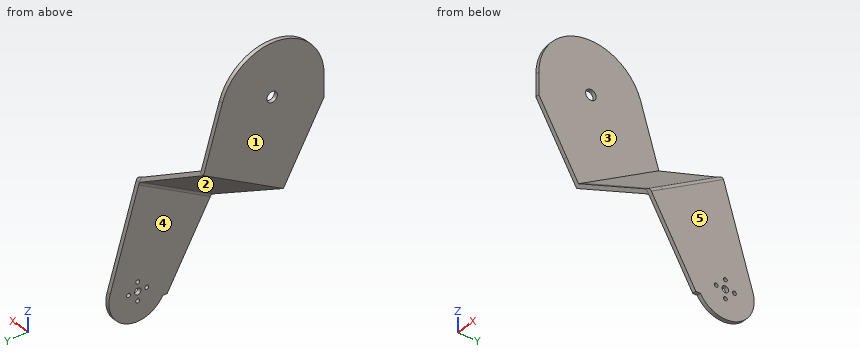
from build123d import *

# Parameters (mm, degrees)
SKETCH_2_R           = 3
SKETCH_2_R_2         = 1.5
SKETCH_2_R_3         = 2.5
EXTRUDE_1_DEPTH      = 3
EXTRUDE_2_DEPTH      = 196
SKETCH_5_R           = 8
CUT_EXTRUDE_1_DEPTH  = 10
SKETCH_6_R           = 4.05
CUT_EXTRUDE_2_DEPTH  = 10
SKETCH_8_R           = 40
EXTRUDE_3_DEPTH      = 3
EXTRUDE_START        = -61
EXTRUDE_4_DEPTH      = 64
EXTRUDE_5_DEPTH      = 3
EXTRUDE_START_2      = -3
EXTRUDE_14_DEPTH     = 3
EXTRUDE_15_DEPTH     = 3
SKETCH_16_R          = 40
EXTRUDE_16_DEPTH     = 3
CUT_EXTRUDE_START    = -20
CUT_EXTRUDE_5_DEPTH  = 20
CUT_EXTRUDE_6_DEPTH  = 20
CUT_EXTRUDE_7_DEPTH  = 3
FILLET_3_R           = 3
FILLET_4_R           = 3
FILLET_5_R           = 3
FILLET_6_R           = 3
SKETCH_22_R          = 7.75
CUT_EXTRUDE_8_DEPTH  = 10
SKETCH_23_R          = 4.05
CUT_EXTRUDE_9_DEPTH  = 10
CUT_EXTRUDE_10_DEPTH = 10
SKETCH_25_W          = 514.702896461
SKETCH_25_H          = 285.568662858
CUT_EXTRUDE_11_DEPTH = 80


# Some blends are built 0.0001 mm under size
with BuildPart() as part:
    # Sketch 2 → Extrude 1 (new body)
    with BuildSketch(Plane(origin=(0, 0, 0), x_dir=(0, 0, -1), z_dir=(1, 0, 0))):
        with BuildLine():
            Line((138.514809283, 84.200667909), (-11.70063651, 38.25042621))
            ThreePointArc((-11.70063651, 38.25042621), (-39.560188627, -5.915359313), (0, -40))
            Line((0, -40), (16.710190716, -40))
            Line((16.710190716, -40), (156.071648789, 40.329376559))
            Line((156.071648789, 40.329376559), (156.071648789, 43.792069046))
            ThreePointArc((156.071648789, 43.792069046), (165.334026038, 71.834783727), (138.514809283, 84.200667909))
        make_face()
        Circle(SKETCH_2_R, mode=Mode.SUBTRACT)
        with Locations((145, 70)):
            Circle(SKETCH_2_R_2, mode=Mode.SUBTRACT)
        with Locations((138, 63)):
            Circle(SKETCH_2_R_2, mode=Mode.SUBTRACT)
        with Locations((145, 56)):
            Circle(SKETCH_2_R_2, mode=Mode.SUBTRACT)
        with Locations((145, 63)):
            Circle(SKETCH_2_R_3, mode=Mode.SUBTRACT)
        with Locations((152, 63)):
            Circle(SKETCH_2_R_2, mode=Mode.SUBTRACT)
    extrude_1 = extrude(amount=EXTRUDE_1_DEPTH)

    # Sketch 4 → Extrude 2 (add)
    with BuildSketch(Plane(origin=(3, 0, 0), x_dir=(0, 0, -1), z_dir=(1, 0, 0))):
        with BuildLine():
            Line((0, -40), (16.710190716, -40))
            Line((16.710190716, -40), (156.071648789, 40.329376559))
            Line((156.071648789, 40.329376559), (156.071648789, 43.792069046))
            Line((156.071648789, 43.792069046), (19.975563357, -34.655113166))
            ThreePointArc((19.975563357, -34.655113166), (10.339136167, -38.640681455), (0, -40))
        make_face()
    extrude(amount=EXTRUDE_2_DEPTH)

    # Mirror 2: Extrude 1 across plane
    add(extrude_1.mirror(Plane(origin=(101, 0, 0), x_dir=(0, 0, 1), z_dir=(1, 0, 0))))

    # Sketch 5 → Cut-Extrude 1 (cut)
    with BuildSketch(Plane(origin=(202, 0, 0), x_dir=(0, 0, -1), z_dir=(1, 0, 0))):
        Circle(SKETCH_5_R)
    extrude(amount=-CUT_EXTRUDE_1_DEPTH, mode=Mode.SUBTRACT)

    # Sketch 6 → Cut-Extrude 2 (cut)
    with BuildSketch(Plane.ZY):
        Circle(SKETCH_6_R)
    extrude(amount=-CUT_EXTRUDE_2_DEPTH, mode=Mode.SUBTRACT)

    # Sketch 9 → Extrude 4 (add)
    with BuildSketch(Plane(origin=(251, 0, 0), x_dir=(0, 0, -1), z_dir=(1, 0, 0)).offset(EXTRUDE_START)):
        with BuildLine():
            Line((0, -40), (16.710190716, -40))
            Line((16.710190716, -40), (53.747942483, -18.651059269))
            Line((53.747942483, -18.651059269), (52.249775231, -16.051925781))
            Line((52.249775231, -16.051925781), (19.975563357, -34.655113166))
            ThreePointArc((19.975563357, -34.655113166), (10.339136167, -38.640681455), (0, -40))
        make_face()
    extrude_4 = extrude(amount=EXTRUDE_4_DEPTH)

    # Sketch 10 → Extrude 5 (add)
    with BuildSketch(Plane(origin=(0, -37.254246654, -21.473730609), x_dir=(1, 0, 0), z_dir=(0, -0.8663778291595938, -0.49938908392225567))):
        Polygon((254, -37.251890328), (254, -57.251890328), (202, -87.274104325), (202, -37.251890328), align=None)
    extrude_5 = extrude(amount=-EXTRUDE_5_DEPTH)



with BuildPart() as body_2:
    # Sketch 8 → Extrude 3 (new body)
    with BuildSketch(Plane(origin=(251, 0, 0), x_dir=(0, 0, -1), z_dir=(1, 0, 0))):
        Circle(SKETCH_8_R)
    extrude(amount=EXTRUDE_3_DEPTH)


with BuildPart() as part_1:
    add(part.part)

    add(body_2.part)  # Extrude 14 merges body 2
    # Sketch 14 → Extrude 14 (add)
    with BuildSketch(Plane(origin=(254, 0, 0), x_dir=(0, 0, -1), z_dir=(1, 0, 0)).offset(EXTRUDE_START_2)):
        with BuildLine():
            Line((-11.70063651, 38.25042621), (35.679778873, 52.743886101))
            Line((35.679778873, 52.743886101), (69.577331814, -6.064144103))
            Line((69.577331814, -6.064144103), (19.975563357, -34.655113166))
            ThreePointArc((19.975563357, -34.655113166), (36.686823541, 15.939792297), (-11.70063651, 38.25042621))
        make_face()
    extrude_14 = extrude(amount=EXTRUDE_14_DEPTH)

    # Sketch 15 → Extrude 15 (add)
    with BuildSketch(Plane(origin=(88.290795719, 76.368648195, -132.490087928), x_dir=(-0.8660254037844362, 0.24969454196113003, -0.4331889145798008), z_dir=(0.5000000000000044, 0.4324836330493111, -0.7503052093278204))):
        Polygon((-191.344507397, -43), (-191.344507397, 27.878041456), (-131.300079402, 20.97393325), (-131.300079402, -43), align=None)
    extrude_15 = extrude(amount=-EXTRUDE_15_DEPTH)

    # Mirror 8: Extrude 15 across plane
    add(extrude_15.mirror(Plane(origin=(101, 0, 0), x_dir=(0, 0, 1), z_dir=(1, 0, 0))))

    # Mirror 10: Extrude 5 across plane
    add(extrude_5.mirror(Plane(origin=(101, 0, 0), x_dir=(0, 0, 1), z_dir=(1, 0, 0))))

    # Mirror 11: Extrude 4 across plane
    add(extrude_4.mirror(Plane(origin=(101, 0, 0), x_dir=(0, 0, 1), z_dir=(1, 0, 0))))

    # Mirror 12: Extrude 14 across plane
    add(extrude_14.mirror(Plane(origin=(101, 0, 0), x_dir=(0, 0, 1), z_dir=(1, 0, 0))))

    # Sketch 16 → Extrude 16 (add)
    with BuildSketch(Plane.ZY.offset(52)):
        Circle(SKETCH_16_R)
    extrude(amount=-EXTRUDE_16_DEPTH)

    # Sketch 17 → Cut-Extrude 5 (cut)
    with BuildSketch(Plane(origin=(202, 0, 0), x_dir=(0, 0, -1), z_dir=(1, 0, 0)).offset(CUT_EXTRUDE_START)):
        with BuildLine():
            Line((-11.120326036, 38.423148607), (61.739147636, 60.715331959))
            Line((61.739147636, 60.715331959), (65.138195736, 61.755085767))
            Line((65.138195736, 61.755085767), (62.037518083, 60.197696416))
            Line((62.037518083, 60.197696416), (92.586691567, 7.198687311))
            Line((92.586691567, 7.198687311), (19.975563357, -34.655113166))
            ThreePointArc((19.975563357, -34.655113166), (-36.806411031, -15.66167638), (-11.120326036, 38.423148607))
        make_face()
    extrude(amount=CUT_EXTRUDE_5_DEPTH, mode=Mode.SUBTRACT)


with BuildPart() as cut_extrude_5_piece_1:
    # of the separate pieces the step leaves, piece 1, a body of its own (cut_extrude_5_pieces)
    add(part_1.part.solids().sort_by_distance((0, 43.792069046, -156.071648789))[0])

    # Sketch 21 → Cut-Extrude 7 (cut)
    with BuildSketch(Plane(origin=(3, 0, 0), x_dir=(0, 0, -1), z_dir=(1, 0, 0))):
        with BuildLine():
            Line((92.586691567, 7.198687311), (62.037518083, 60.197696416))
            Line((62.037518083, 60.197696416), (65.138195736, 61.755085767))
            Line((65.138195736, 61.755085767), (61.739147636, 60.715331959))
            Line((61.739147636, 60.715331959), (-11.70063651, 38.25042621))
            ThreePointArc((-11.70063651, 38.25042621), (-36.686823541, -15.939792297), (19.975563357, -34.655113166))
            Line((19.975563357, -34.655113166), (92.586691567, 7.198687311))
        make_face()
    extrude(amount=-CUT_EXTRUDE_7_DEPTH, mode=Mode.SUBTRACT)

    # Fillet 3
    fillet_3_edges = [cut_extrude_5_piece_1.edges().sort_by_distance(p)[0] for p in [
        (3, 33.698191863, -77.312104825),
    ]]
    fillet(fillet_3_edges, radius=FILLET_3_R - 0.0001)  # a hair under: the kernel refuses the full size

    # Fillet 4
    fillet_4_edges = [cut_extrude_5_piece_1.edges().sort_by_distance(p)[0] for p in [
        (199, 33.698191863, -77.312104825),
    ]]
    fillet(fillet_4_edges, radius=FILLET_4_R - 0.0001)  # a hair under: the kernel refuses the full size

    # Fillet 5
    # the kernel refuses this fillet: 3 mm, written as the material it adds along each edge
    with BuildSketch(Plane(origin=(202, 65.506611814, -62.97577757), x_dir=(0, 0.49938908392225534, -0.8663778291595939), z_dir=(0, -0.866377829159594, -0.4993890839222554))) as fillet_5_piece_1_section:
        with BuildLine():
            CenterArc((FILLET_5_R * 0.57735026919, FILLET_5_R), FILLET_5_R, 210, 60)
            Line((-FILLET_5_R * 0.288675134595, FILLET_5_R * 0.5), (0, 0))
            Line((0, 0), (FILLET_5_R * 0.57735026919, 0))
        make_face()
    fillet_5_piece_1 = extrude(amount=68.304060269, mode=Mode.PRIVATE)
    fillet_5_piece_1 = split(fillet_5_piece_1, bisect_by=Plane(origin=(202.325553984, 63.906694987, -72.171998522), z_dir=(0, -0.9562606552534866, -0.2925159127537726)), keep=Keep.TOP, mode=Mode.PRIVATE)
    fillet_5_piece_1 = split(fillet_5_piece_1, bisect_by=Plane(origin=(199.177617764, 62.412552566, -67.072312804), z_dir=(0.09892666816624712, -0.8892295154916122, -0.44663674625368427)), keep=Keep.TOP, mode=Mode.PRIVATE)
    add(fillet_5_piece_1)

    # Fillet 6
    # the kernel refuses this fillet: 3 mm, written as the material it adds along each edge
    with BuildSketch(Plane(origin=(0, 6.329488355, -97.086079656), x_dir=(2.017234182721707e-14, 0.49938908392225534, -0.8663778291595939), z_dir=(0, 0.8663778291595939, 0.4993890839222554))) as fillet_6_piece_1_section:
        with BuildLine():
            CenterArc((FILLET_6_R * 0.57735026919, FILLET_6_R), FILLET_6_R, 210, 60)
            Line((-FILLET_6_R * 0.288675134595, FILLET_6_R * 0.5), (0, 0))
            Line((0, 0), (FILLET_6_R * 0.57735026919, 0))
        make_face()
    fillet_6_piece_1 = extrude(amount=68.304060269, mode=Mode.PRIVATE)
    fillet_6_piece_1 = split(fillet_6_piece_1, bisect_by=Plane(origin=(-0.325553984, 63.906694987, -72.171998522), z_dir=(0, -0.9562606552534866, -0.2925159127537726)), keep=Keep.TOP, mode=Mode.PRIVATE)
    fillet_6_piece_1 = split(fillet_6_piece_1, bisect_by=Plane(origin=(2.822382236, 62.412552566, -67.072312804), z_dir=(-0.09892666816624712, -0.8892295154916122, -0.44663674625368427)), keep=Keep.TOP, mode=Mode.PRIVATE)
    add(fillet_6_piece_1)

    # Sketch 22 → Cut-Extrude 8 (cut)
    with BuildSketch(Plane(origin=(254, 0, 0), x_dir=(0, 0, -1), z_dir=(1, 0, 0))):
        Circle(SKETCH_22_R)
    extrude(amount=-CUT_EXTRUDE_8_DEPTH, mode=Mode.SUBTRACT)

    # Sketch 23 → Cut-Extrude 9 (cut)
    with BuildSketch(Plane.ZY.offset(52)):
        Circle(SKETCH_23_R)
    extrude(amount=-CUT_EXTRUDE_9_DEPTH, mode=Mode.SUBTRACT)

    # Sketch 24 → Cut-Extrude 10 (cut)
    with BuildSketch(Plane(origin=(0, -37.254246654, -21.473730609), x_dir=(1, 0, 0), z_dir=(0, -0.8663778291595938, -0.49938908392225567))):
        with BuildLine():
            Line((-49, 40), (-49, -55.51983952))
            Line((-49, -55.51983952), (0, -83.81000271))
            ThreePointArc((0, -83.81000271), (2.121320344, -84.688682367), (3, -86.81000271))
            Line((3, -86.81000271), (3, -87.274104325))
            Line((3, -87.274104325), (3, -179.256683584))
            Line((3, -179.256683584), (199, -179.256683584))
            Line((199, -179.256683584), (199, -87.274104325))
            Line((199, -87.274104325), (199, -86.81000271))
            ThreePointArc((199, -86.81000271), (199.878679656, -84.688682367), (202, -83.81000271))
            Line((202, -83.81000271), (251, -55.51983952))
            Line((251, -55.51983952), (251, 40))
            Line((251, 40), (-49, 40))
        make_face()
    extrude(amount=-CUT_EXTRUDE_10_DEPTH, mode=Mode.SUBTRACT)


with BuildPart() as cut_extrude_5_piece_2:
    # of the separate pieces the step leaves, piece 2, a body of its own (cut_extrude_5_pieces)
    add(part_1.part.solids().sort_by_distance((202, 60.715331959, -61.739147636))[0])

    # Sketch 18 → Cut-Extrude 6 (cut)
    with BuildSketch(Plane(origin=(0, 38.25042621, 11.70063651), x_dir=(1, 0, 0), z_dir=(0, 0.9562606552534866, 0.2925159127537726))):
        Polygon((199, 76.798918519), (202, 76.932821805), (202, 0), (199, 0), align=None)
    extrude(amount=-CUT_EXTRUDE_6_DEPTH, mode=Mode.SUBTRACT)


with BuildPart() as cut_extrude_10_piece_1:
    # of the separate pieces the step leaves, piece 1, a body of its own (cut_extrude_10_pieces)
    add(cut_extrude_5_piece_1.part.solids().sort_by_distance((-1.5, 5.897004722, -96.335774447))[0])


with BuildPart() as cut_extrude_10_piece_2:
    # of the separate pieces the step leaves, piece 2, a body of its own (cut_extrude_10_pieces)
    add(cut_extrude_5_piece_1.part.solids().sort_by_distance((199, 6.097721075, -96.683992306))[0])

    # Sketch 25 → Cut-Extrude 11 (cut)
    with BuildSketch(Plane(origin=(254, 0, 0), x_dir=(0, 0, -1), z_dir=(1, 0, 0))):
        with Locations((-76.2896691, 93.84361465)):
            Rectangle(SKETCH_25_W, SKETCH_25_H)
    extrude(amount=-CUT_EXTRUDE_11_DEPTH, mode=Mode.SUBTRACT)


solid = cut_extrude_10_piece_1.part
Could you check a few things on this model? Use its own coordinates, in mm. Face numbers are marked on the shaded views. A direction names the side the tool comes from. Round coordinates to 2 decimals unless told otherwise and drop trailing zeros. Order: outer loops, then holes, each group sorted by start corner. A loop starts at its lowest first (then second) coordinate and runs counter-clockwise, first axis right, second up.
(1) Imagine slicing it at C-C (z = -103.5). Write out the boundary of the cut face in (x, y).
Response values:
outline: (0, 10.03) - (3, 10.03) - (3, 73.49) - (0, 73.49) - close
(2) Which directions (+Z, -Z, +X, -X, +Y, -Y) give clear straight access to the entire face, cutting with the end or side of a thin tool? Please do the marked faces 3, 4 and 5.
Response values:
face 3: +Z, +X, -Y
face 4: -Z, -X, +Y
face 5: +Z, -Z, +X, +Y, -Y
(3) Imagine slicing it at A-A (y = 0). Write out the boundary of the cut face in (x, z).
Response values:
outline: (-52, -66.08) - (-21.95, -86.11) - (-15.95, -86.11) - (-49, -64.08) - (-49, -4.05) - (-52, -4.05) - close; (-52, 4.05) - (-49, 4.05) - (-49, 40) - (-52, 40) - close
(4) Please list where these lines run through material, in increasing order: line 1 along Y through (x, z) = (2.3, -145); line 2 along X through (y, z) = (27, -119.5); line 3 along X through (y, z) = (23, 27.5).
Response values:
line 1: y = 33.95 to 54.5, 57.5 to 60.5, 65.5 to 68.5, 71.5 to 85.17
line 2: x = 0 to 3
line 3: x = -52 to -49
(5) Imagine slicing it at D-D (x = -35). Write out the boundary of the cut face in (y, z).
Response values:
outline: (-5.49, -76.58) - (-3.76, -79.58) - (55.69, -45.31) - (54.13, -42.21) - close
(6) I'm going to push flat-ended pins straight in: pin 1 (5 mm diameter, centred on y = 63, z = -138, fed in from +X); pin 2 (3 mm diameter, centred on y = 63, z = -145, fed in from +X); pin 3 (3.5 mm diameter, centred on y = 63, z = -152, fed in from -X); pin 4 (4 mm diameter, centred on x = -38, y = -7.5, fed in from -Z). Where does each tip first touch, or does it pass through?
Response values:
pin 1: stops at x = 3
pin 2: passes through
pin 3: stops at x = 0
pin 4: stops at z = -76.56
(7) Imagine slicing it at B-B (x = -14). Write out the boundary of the cut face in (y, z), plus the area to 3 significant figures.
Response values:
outline: (0.56, -87.08) - (2.29, -90.08) - (59.33, -57.21) - (57.77, -54.11) - close
area: 228 mm2
(8) If we mould it in two halves opening along Y, with no side actions, what happens to the marked faces 1 and 2? For each: released by +Y, released by -Y, zero draft, split by the parting line, or undercut.
Response values:
face 1: zero draft
face 2: released by +Y
